Geometry: final body of the model. Coordinates: model frame, mm. A direction names the side the tool comes from. Give positions to 0.01 mm unless a question says otherwise; leave off trailing zeros. Write each loop counter-clockwise with the first axis right and the second up, starting at its lowest first coordinate (ties: lowest second). Pieces come first, ordered by that corner, then holes. Notation, with made-up numbers: (41.5, 55.25) -> (55.5, 55.25) arc R21 cw to (55.5, 73.25) -> close; hole circle Ø6 at (52, -38). An arc over 180 degrees is marked (long way). Answer in a Markdown table with one row per item. Add a question column.
Item 1: Access query for faces 1 (the cylindrical face through (1.21, 74.57, 1.53)), 2 (the flat face through (-39, 48, 0)). Directions: +Z, -Z, +X, -X, +Y, -Y. A direction counts if a zero-diameter tool reaches every point of the face in a straight line with its end or side. Return the directions, or none.
Item 2: Section query A-A on x = 0. Output: boundary loops of the cut face in (y, z).
Item 3: Section query B-B on y = 0. Output: boundary loops of the cut face in (x, z), plus the area to 3 significant figures.
Item 4: Section query D-D on x = 73.5. Output: boundary loops of the cut face in (y, z).
Item 5: First-contact query: P1, Ø3, axis at y = 29.5, z = -9, coming from the +X side; P2, Ø10, axis at x = -61, y = 55, coming from the -Z side; P3, Ø8, axis at x = 25.5, y = -26, coming from the -Z side. Flat tips, straight axial feed; report the tip coordinate or a pass-through.
Item 6: Material intervals for probe 1 along X at (y, z) = (-2, 39); probe 2 along Y at (x, z) = (0, 19.5); probe 3 along Z at (x, y) = (55, -57.5), sorted ascending. Write a range as from..to.
Item 7: Section query C-C on z = 34. Output: boundary loops of the cut face in (x, y), plus the area to 3 significant figures.
```python
from build123d import *

# Parameters (mm, degrees)
F0_W     = 182.3617219925
F0_H     = 152.0290374756
F1_DEPTH = 172.974
F2_R     = 55.9466772096
F3_DEPTH = 54.61
F4_R     = 41.7280141722
F5_DEPTH = 271.272
F6_R     = 5.08


with BuildPart() as f1:
    # F0 (on Top) → F1 (new body)
    with BuildSketch(Plane.XY):
        Rectangle(F0_W, F0_H)
    extrude(amount=F1_DEPTH)

    # F2 (on Top) → F3 (join)
    with BuildSketch(Plane.XY):
        Circle(F2_R)
    extrude(amount=-F3_DEPTH)

    # F4 (on face) → F5 (cut)
    with BuildSketch(Plane(origin=(0, 0, -54.61), x_dir=(1, 0, 0), z_dir=(0, 0, -1))):
        Circle(F4_R)
    extrude(amount=-F5_DEPTH, mode=Mode.SUBTRACT)

    # F6
    f6_edges = [f1.edges().sort_by_distance(p)[0] for p in [
        (91.180861, 76.014519, 86.487),
        (-91.180861, 76.014519, 86.487),
        (0, 76.014519, 0),
        (0, 76.014519, 172.974),
        (91.180861, 0, 0),
        (-91.180861, 0, 0),
        (0, -76.014519, 0),
        (-55.946677, 0, 0),
        (-91.180861, -76.014519, 86.487),
        (-91.180861, 0, 172.974),
        (55.946677, 0, -27.305),
        (-55.946677, 0, -54.61),
        (-41.728014, 0, -54.61),
        (41.728014, 0, 59.182),
        (-41.728014, 0, 172.974),
        (91.180861, 0, 172.974),
        (91.180861, -76.014519, 86.487),
        (0, -76.014519, 172.974),
    ]]
    fillet(f6_edges, radius=F6_R)


solid = f1.part
```
Findings below:
| question | item | result |
|---|---|---|
| 1 | face 1 | -Z, +X, -X, +Y |
| 1 | face 2 | -Z |
| 2 | outline | (-76.01, 5.08) arc R5.08 ccw to (-70.93, 0) -> (-61.03, 0) arc R5.08 cw to (-55.95, -5.08) -> (-55.95, -49.53) arc R5.08 ccw to (-50.87, -54.61) -> (-46.81, -54.61) arc R5.08 ccw to (-41.73, -49.53) -> (-41.73, 167.89) arc R5.08 ccw to (-46.81, 172.97) -> (-70.93, 172.97) arc R5.08 ccw to (-76.01, 167.89) -> close; (41.73, -49.53) arc R5.08 ccw to (46.81, -54.61) -> (50.87, -54.61) arc R5.08 ccw to (55.95, -49.53) -> (55.95, -5.08) arc R5.08 cw to (61.03, 0) -> (70.93, 0) arc R5.08 ccw to (76.01, 5.08) -> (76.01, 167.89) arc R5.08 ccw to (70.93, 172.97) -> (46.81, 172.97) arc R5.08 ccw to (41.73, 167.89) -> close |
| 3 | outline | (-91.18, 5.08) arc R5.08 ccw to (-86.1, 0) -> (-61.03, 0) arc R5.08 cw to (-55.95, -5.08) -> (-55.95, -49.53) arc R5.08 ccw to (-50.87, -54.61) -> (-46.81, -54.61) arc R5.08 ccw to (-41.73, -49.53) -> (-41.73, 167.89) arc R5.08 ccw to (-46.81, 172.97) -> (-86.1, 172.97) arc R5.08 ccw to (-91.18, 167.89) -> close; (41.73, -49.53) arc R5.08 ccw to (46.81, -54.61) -> (50.87, -54.61) arc R5.08 ccw to (55.95, -49.53) -> (55.95, -5.08) arc R5.08 cw to (61.03, 0) -> (86.1, 0) arc R5.08 ccw to (91.18, 5.08) -> (91.18, 167.89) arc R5.08 ccw to (86.1, 172.97) -> (46.81, 172.97) arc R5.08 ccw to (41.73, 167.89) -> close |
| 3 | area | 18,600 mm^2 |
| 4 | outline | (-76.01, 5.08) arc R5.08 ccw to (-70.93, 0) -> (70.93, 0) arc R5.08 ccw to (76.01, 5.08) -> (76.01, 167.89) arc R5.08 ccw to (70.93, 172.97) -> (-70.93, 172.97) arc R5.08 ccw to (-76.01, 167.89) -> close |
| 5 | P1 | stops at x = 48.44 |
| 5 | P2 | stops at z = 0 |
| 5 | P3 | passes through |
| 6 | probe 1 | x = -91.18..-41.68, 41.68..91.18 |
| 6 | probe 2 | y = -76.01..-41.73, 41.73..76.01 |
| 6 | probe 3 | z = 0..172.97 |
| 7 | outline | (-91.18, -70.93) arc R5.08 ccw to (-86.1, -76.01) -> (86.1, -76.01) arc R5.08 ccw to (91.18, -70.93) -> (91.18, 70.93) arc R5.08 ccw to (86.1, 76.01) -> (-86.1, 76.01) arc R5.08 ccw to (-91.18, 70.93) -> close; hole circle Ø83.46 at (0, 0) |
| 7 | area | 22,200 mm^2 |
